Work out the finished part from the listing and answer in its coordinate system (mm). Round coordinates to 2 decimals unless told otherwise and drop trailing zeros. Loops run counter-clockwise (first coordinate to the right, second up) from the corner with the lowest first, then second, coordinate; pieces in that order, holes last. Notation, with made-up numbers: (58.5, 55.25) - (103.5, 55.25) arc R17 ccw to (103.5, 70.25) - close; hole circle Ø8 at (64.25, -24). An arc over 180 degrees is marked (long way). Return JSON: item names as keys, results as strings.
from build123d import *

# Parameters (mm, degrees)
SKETCH_1_W      = 128
SKETCH_1_H      = 100
SKETCH_1_R      = 1.55
EXTRUDE_1_DEPTH = 3


with BuildPart() as part:
    # 草图1 → 凸台-拉伸1 (new body)
    with BuildSketch(Plane(origin=(0, 0, 0), x_dir=(1, 0, 0), z_dir=(0, 1, 0))):
        Rectangle(SKETCH_1_W, SKETCH_1_H)
        with Locations(Location((-60, -46, 0), (0, 0, 270))):
            Circle(SKETCH_1_R, mode=Mode.SUBTRACT)
        with Locations(Location((-37, -46, 0), (0, 0, 270))):
            Circle(SKETCH_1_R, mode=Mode.SUBTRACT)
        with Locations(Location((-37, -34, 0), (0, 0, 270))):
            Circle(SKETCH_1_R, mode=Mode.SUBTRACT)
        with Locations(Location((-60, -34, 0), (0, 0, 270))):
            Circle(SKETCH_1_R, mode=Mode.SUBTRACT)
        with Locations(Location((-37, -10, 0), (0, 0, 270))):
            Circle(SKETCH_1_R, mode=Mode.SUBTRACT)
        with Locations(Location((-37, -22, 0), (0, 0, 270))):
            Circle(SKETCH_1_R, mode=Mode.SUBTRACT)
        with Locations(Location((-60, -10, 0), (0, 0, 270))):
            Circle(SKETCH_1_R, mode=Mode.SUBTRACT)
        with Locations(Location((-60, -22, 0), (0, 0, 270))):
            Circle(SKETCH_1_R, mode=Mode.SUBTRACT)
        with Locations(Location((60, -34, 0), (0, 0, 90))):
            Circle(SKETCH_1_R, mode=Mode.SUBTRACT)
        with Locations(Location((60, -46, 0), (0, 0, 90))):
            Circle(SKETCH_1_R, mode=Mode.SUBTRACT)
        with Locations(Location((37, -46, 0), (0, 0, 90))):
            Circle(SKETCH_1_R, mode=Mode.SUBTRACT)
        with Locations(Location((37, -34, 0), (0, 0, 90))):
            Circle(SKETCH_1_R, mode=Mode.SUBTRACT)
        with Locations(Location((60, -22, 0), (0, 0, 90))):
            Circle(SKETCH_1_R, mode=Mode.SUBTRACT)
        with Locations(Location((37, -22, 0), (0, 0, 90))):
            Circle(SKETCH_1_R, mode=Mode.SUBTRACT)
        with Locations(Location((37, -10, 0), (0, 0, 90))):
            Circle(SKETCH_1_R, mode=Mode.SUBTRACT)
        with Locations(Location((60, -10, 0), (0, 0, 90))):
            Circle(SKETCH_1_R, mode=Mode.SUBTRACT)
        with Locations(Location((60, 10, 0), (0, 0, 270))):
            Circle(SKETCH_1_R, mode=Mode.SUBTRACT)
        with Locations(Location((37, 10, 0), (0, 0, 270))):
            Circle(SKETCH_1_R, mode=Mode.SUBTRACT)
        with Locations(Location((37, 22, 0), (0, 0, 270))):
            Circle(SKETCH_1_R, mode=Mode.SUBTRACT)
        with Locations(Location((60, 22, 0), (0, 0, 270))):
            Circle(SKETCH_1_R, mode=Mode.SUBTRACT)
        with Locations(Location((60, 34, 0), (0, 0, 270))):
            Circle(SKETCH_1_R, mode=Mode.SUBTRACT)
        with Locations(Location((60, 46, 0), (0, 0, 270))):
            Circle(SKETCH_1_R, mode=Mode.SUBTRACT)
        with Locations(Location((37, 34, 0), (0, 0, 270))):
            Circle(SKETCH_1_R, mode=Mode.SUBTRACT)
        with Locations(Location((37, 46, 0), (0, 0, 270))):
            Circle(SKETCH_1_R, mode=Mode.SUBTRACT)
        with Locations(Location((-60, 46, 0), (0, 0, 90))):
            Circle(SKETCH_1_R, mode=Mode.SUBTRACT)
        with Locations(Location((-37, 46, 0), (0, 0, 90))):
            Circle(SKETCH_1_R, mode=Mode.SUBTRACT)
        with Locations(Location((-37, 34, 0), (0, 0, 90))):
            Circle(SKETCH_1_R, mode=Mode.SUBTRACT)
        with Locations(Location((-60, 34, 0), (0, 0, 90))):
            Circle(SKETCH_1_R, mode=Mode.SUBTRACT)
        with Locations(Location((-60, 22, 0), (0, 0, 90))):
            Circle(SKETCH_1_R, mode=Mode.SUBTRACT)
        with Locations(Location((-37, 22, 0), (0, 0, 90))):
            Circle(SKETCH_1_R, mode=Mode.SUBTRACT)
        with Locations(Location((-37, 10, 0), (0, 0, 90))):
            Circle(SKETCH_1_R, mode=Mode.SUBTRACT)
        with Locations(Location((-60, 10, 0), (0, 0, 90))):
            Circle(SKETCH_1_R, mode=Mode.SUBTRACT)
    extrude(amount=EXTRUDE_1_DEPTH)


solid = part.part
1) Find the intervals of material crossed by L1, parallel to X at y = 1.65, z = -34; L2, parallel to X at y = 1.85, z = 35, in increasing order.
Verdict:
{"L1": "x = -64 to -61.55, -58.45 to -38.55, -35.45 to 35.45, 38.55 to 58.45, 61.55 to 64", "L2": "x = -64 to -61.18, -58.82 to -38.18, -35.82 to 35.82, 38.18 to 58.82, 61.18 to 64"}
2) Section B-B (y = 1.8) is taken. Count the separate pieces of the cut face and the enclosed holes in it, and give its area (3 significant figures).
Verdict:
{"separate pieces": "1", "enclosed holes": "32", "area": "12,600 mm2"}
3) Section A-A (z = 22) is taken. Give the vertices of the cut face in (x, y).
Verdict:
{"outline": "(-64, 0) - (-61.55, 0) - (-61.55, 3) - (-64, 3) - close; (-58.45, 0) - (-38.55, 0) - (-38.55, 3) - (-58.45, 3) - close; (-35.45, 0) - (35.45, 0) - (35.45, 3) - (-35.45, 3) - close; (38.55, 0) - (58.45, 0) - (58.45, 3) - (38.55, 3) - close; (61.55, 0) - (64, 0) - (64, 3) - (61.55, 3) - close"}
4) Determine the mould class of faces 1 (the cylindrical face through (61.537, 1.479, -10.202)), 2 (the flat face through (64, 1, 1)) for opening direction Z: pulls with the +Z half, pulls with the -Z half, needs draft (parallel to the pull), parting line crosses it, or undercut.
Verdict:
{"face 1": "undercut", "face 2": "needs draft"}
5) A flat-ended cylindrical pin translates along its axis: pin 1 (3 mm diameter, centred on x = 60, z = 10, fed in from -Y). Find the tip coordinate at first contact, or state that the pin passes through.
Verdict:
{"pin 1": "passes through"}
